The figure shows three views and two pictorial views of one solid part (mm, origin at its lowest corner). Answer the questions. A direction names the side the tool comes from. Give positions to 0.01 mm unless a question says otherwise; leave off trailing zeros. Loops run counter-clockwise (first coordinate to the right, second up) from the corner with the lowest first, then second, coordinate; pieces in that order, holes last. Notation, with made-up numbers: (36.5, 4) - (76.5, 4) arc R24 cw to (76.5, 21) - close; hole circle Ø6 at (56, 20.25). An arc over 180 degrees is marked (long way). One line per question, with ' | ' between items.
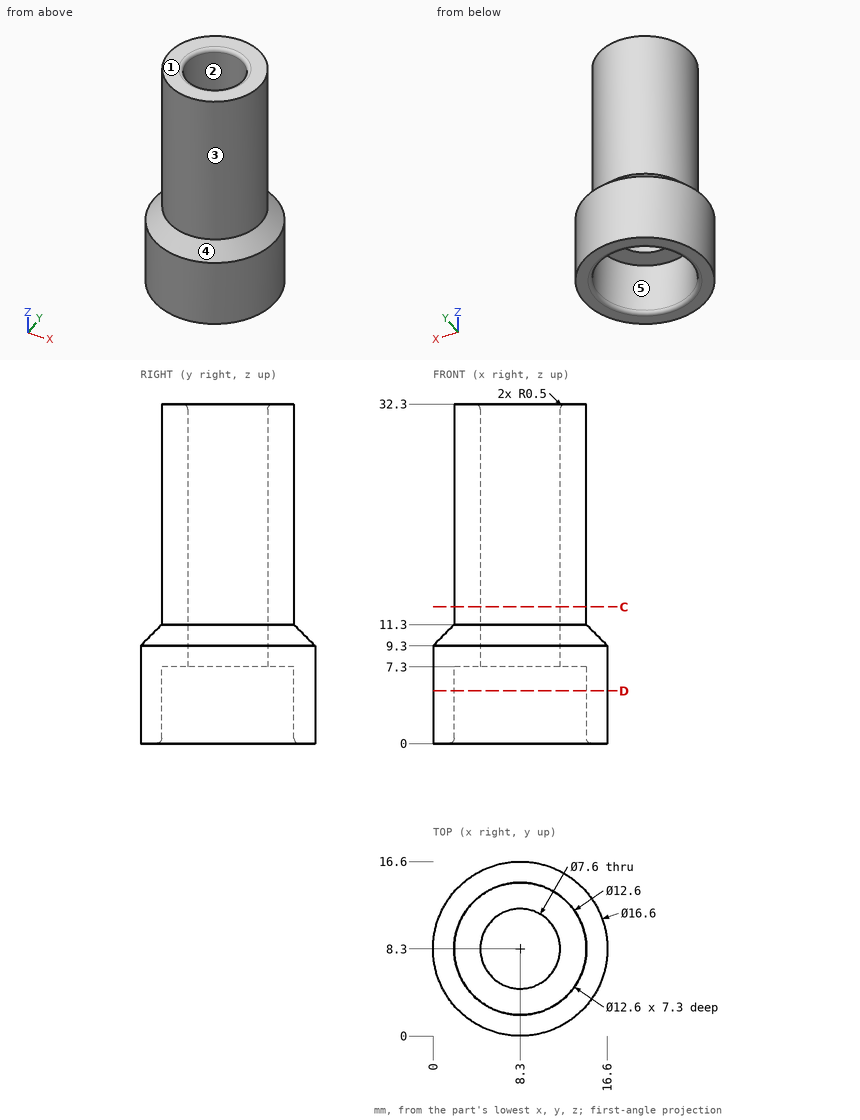
1. Which of the six approach directions +Z, -Z, +X, -X, +Y, -Y give full straight-line access (tool end or side, diameter ignored) to the marked faces 4 and 5?
Evaluation:
face 4: +Z | face 5: -Z
2. Find section C-C on z = 13. Write down the section's boundary in (x, y), then the cut area to 3 significant figures.
Evaluation:
outline: circle Ø12.6 at (8.3, 8.3); hole circle Ø7.6 at (8.3, 8.3) | area: 79.3 mm2
3. Flat-ended cylindrical pins translate along their axes: pin 1 (1 mm diameter, centred on x = 14, y = 7.5, fed in from -Z); pin 2 (1.5 mm diameter, centred on x = 10.5, z = 7, fed in from -Y); pin 3 (4 mm diameter, centred on y = 4.5, z = 24.5, fed in from -X). Find the tip coordinate at first contact, or state that the pin passes through.
Evaluation:
pin 1: z = 7.3 | pin 2: y = 0.13 | pin 3: x = 2.26
4. Consider L1, parallel to X at y = 8.3, z = 4.75; L2, parallel to Y at x = 8.3, z = 25.5; L3, parallel to Z at x = 4.75, y = 6. Determine where each line is inside the solid, lowest interval first.
Evaluation:
L1: 0 to 2, 14.6 to 16.6 | L2: 2 to 4.5, 12.1 to 14.6 | L3: 7.3 to 32.3
5. Determine the mould class of the marked faces 1, 2 and 3 for opening direction X: +X half, -X half, draft (parallel to the pull), parting line (faces both ways), or undercut.
Evaluation:
face 1: draft | face 2: undercut | face 3: parting line
6. Find section D-D on z = 5. Write down the section's boundary in (x, y).
Evaluation:
outline: circle Ø16.6 at (8.3, 8.3); hole circle Ø12.6 at (8.3, 8.3)
